Can you work these out from the model? Positions are in its coordinate system, mm. Round coordinates to 2 decimals unless told otherwise and drop trailing zeros. Order: outer loops, then holes, each group sorted by start corner. A loop starts at its lowest first (then second) coordinate and runs counter-clockwise, first axis right, second up.
Q1. If we section it at A-A (y = 0): Please give me the cut outline in (x, z), plus the area to 3 significant figures.
Q2. If I drill on line 1 (X direction, y = 11.5, z = 4.75); line 2 (Y direction, x = 1066.8, z = 3.75); line 3 (Y direction, x = 728, z = 9.75), over which ranges is the centre line in solid material (lowest first)?
Q3. If we section it at B-B (z = 3): Please give me the cut outline in (x, y), plus the area to 3 significant figures.
Q4. Will these pins go through, and if not, where does the flat tip stop? P1, Ø5, axis at y = 7.5, z = 6.5, coming from the -X side; P2, Ø1, axis at y = -1, z = 5, coming from the -X side.
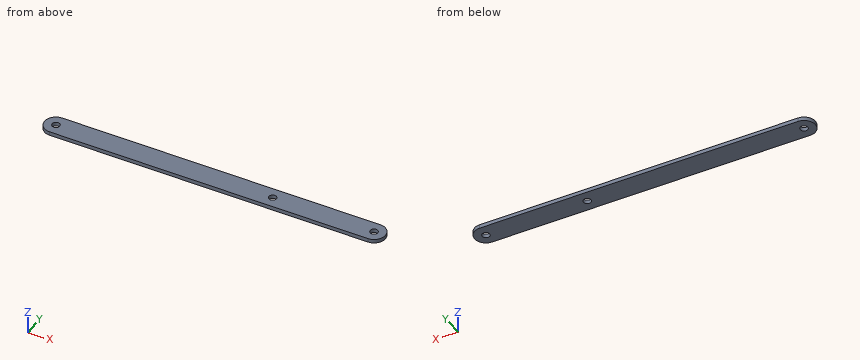
from build123d import *

# Parameters (mm, degrees)
SKETCH2_R           = 12.7
BOSS_EXTRUDE1_DEPTH = 12.7
SKETCH3_R           = 12.7
CUT_EXTRUDE1_DEPTH  = 13.7


with BuildPart() as part:
    # Sketch2 → Boss-Extrude1 (new body)
    with BuildSketch(Plane.XY):
        with BuildLine():
            Line((0, 38.1), (1066.8, 38.1))
            ThreePointArc((1066.8, 38.1), (1104.9, 0), (1066.8, -38.1))
            Line((1066.8, -38.1), (0, -38.1))
            ThreePointArc((0, -38.1), (-38.1, 0), (0, 38.1))
        make_face()
        Circle(SKETCH2_R, mode=Mode.SUBTRACT)
        with Locations((1066.8, 0)):
            Circle(SKETCH2_R, mode=Mode.SUBTRACT)
    extrude(amount=BOSS_EXTRUDE1_DEPTH)

    # Sketch3 → Cut-Extrude1 (cut, through all)
    with BuildSketch(Plane.XY.offset(12.7)):
        with Locations((726.772091625, 0)):
            Circle(SKETCH3_R)
    extrude(amount=-CUT_EXTRUDE1_DEPTH, mode=Mode.SUBTRACT)


solid = part.part
Solution:
1. outline: (-38.1, 0) - (-12.7, 0) - (-12.7, 12.7) - (-38.1, 12.7) - close; (12.7, 0) - (714.07, 0) - (714.07, 12.7) - (12.7, 12.7) - close; (739.47, 0) - (1054.1, 0) - (1054.1, 12.7) - (739.47, 12.7) - close; (1079.5, 0) - (1104.9, 0) - (1104.9, 12.7) - (1079.5, 12.7) - close
1. area: 13,500 mm2
2. line 1: x = -36.32 to -5.39, 5.39 to 721.38, 732.16 to 1061.41, 1072.19 to 1103.12
2. line 2: y = -38.1 to -12.7, 12.7 to 38.1
2. line 3: y = -38.1 to -12.64, 12.64 to 38.1
3. outline: (0, -38.1) - (1066.8, -38.1) arc R38.1 ccw to (1066.8, 38.1) - (0, 38.1) arc R38.1 ccw to start; hole circle Ø25.4 at (0, 0); hole circle Ø25.4 at (726.77, 0); hole circle Ø25.4 at (1066.8, 0)
3. area: 84,300 mm2
4. P1: stops at x = -37.77
4. P2: stops at x = -38.1
